from build123d import *

# Parameters (mm, degrees)
F1_DEPTH = 6.35


with BuildPart() as f1:
    # F0 (on Top) → F1 (new body)
    with BuildSketch(Plane.XY):
        with BuildLine():
            Line((-51.2445, 0), (-48.26, 0))
            ThreePointArc((-48.26, 0), (-54.61, 6.35), (-60.96, 0))
            Line((-60.96, 0), (-57.9755, 0))
            ThreePointArc((-57.9755, 0), (-54.61, 3.3655), (-51.2445, 0))
        make_face()
        with BuildLine():
            ThreePointArc((-60.96, 0), (-54.61, -6.35), (-48.26, 0))
            Line((-48.26, 0), (-51.2445, 0))
            ThreePointArc((-51.2445, 0), (-54.61, -3.3655), (-57.9755, 0))
            Line((-57.9755, 0), (-60.96, 0))
        make_face()
        with BuildLine():
            ThreePointArc((-34.1249732601, -34.1249732601), (-44.586426239, -18.4683024459), (-48.26, 0))
            ThreePointArc((-48.26, 0), (-54.61, -6.35), (-60.96, 0))
            ThreePointArc((-60.96, 0), (-37.1100967124, -48.3628196242), (15.7776089894, -58.8828383706))
            ThreePointArc((15.7776089894, -58.8828383706), (12.4119310117, -58.8612144651), (9.5300837025, -57.1224758622))
            ThreePointArc((9.5300837025, -57.1224758622), (-17.6688931256, -55.1507929201), (-40.9499679121, -40.9499679121))
            ThreePointArc((-40.9499679121, -40.9499679121), (-40.9499679121, -36.2802347291), (-36.2802347291, -36.2802347291))
            Line((-36.2802347291, -36.2802347291), (-34.1249732601, -34.1249732601))
        make_face()
        with BuildLine():
            ThreePointArc((8.1381651285, -50.6584754246), (9.8124734412, -48.096685942), (12.4906071166, -46.6155803767))
            ThreePointArc((12.4906071166, -46.6155803767), (-12.4906071166, -46.6155803767), (-34.1249732601, -34.1249732601))
            Line((-34.1249732601, -34.1249732601), (-36.2802347291, -36.2802347291))
            ThreePointArc((-36.2802347291, -36.2802347291), (-15.8011857696, -48.8142744725), (8.1381651285, -50.6584754246))
        make_face()
        with BuildLine():
            ThreePointArc((20.484108053, -52.7492093736), (17.9997431273, -47.7114156628), (12.4906071166, -46.6155803767))
            Line((12.4906071166, -46.6155803767), (13.2794875661, -49.5597222952))
            ThreePointArc((13.2794875661, -49.5597222952), (16.1442382916, -50.129556644), (17.436108053, -52.7492093736))
            ThreePointArc((17.436108053, -52.7492093736), (16.7537607827, -54.7593396122), (14.98872854, -55.9386964521))
            Line((14.98872854, -55.9386964521), (15.7776089894, -58.8828383706))
            ThreePointArc((15.7776089894, -58.8828383706), (19.1719017639, -56.6148444479), (20.484108053, -52.7492093736))
        make_face()
        with BuildLine():
            Line((13.2794875661, -49.5597222952), (12.4906071166, -46.6155803767))
            ThreePointArc((12.4906071166, -46.6155803767), (9.8124734412, -48.096685942), (8.1381651285, -50.6584754246))
            ThreePointArc((8.1381651285, -50.6584754246), (10.7229089499, -50.1749946453), (13.2794875661, -49.5597222952))
        make_face()
        with BuildLine():
            ThreePointArc((9.5300837025, -57.1224758622), (12.4119310117, -58.8612144651), (15.7776089894, -58.8828383706))
            Line((15.7776089894, -58.8828383706), (14.98872854, -55.9386964521))
            ThreePointArc((14.98872854, -55.9386964521), (12.2736861565, -56.5964342705), (9.5300837025, -57.1224758622))
        make_face()
    extrude(amount=-F1_DEPTH)


solid = f1.part
Check sheet for the modelled part. Datum: model origin and axes. Units: mm. Round coordinates to 2 decimals unless told otherwise and drop trailing zeros. Write each loop counter-clockwise with the first axis right and the second up, starting at its lowest first coordinate (ties: lowest second). Pieces come first, ordered by that corner, then holes. Notation, with made-up numbers: (8, 1) -> (14, 1) arc R15 ccw to (14, 18) -> close; hole circle Ø1 at (56, 21). An arc over 180 degrees is marked (long way). Answer as CSV lines item,"result". Start each with the question number.
1) Section check B-B on z = -3. Enter the section's corners in (x, y), and give its area (3 significant figures).
2) Section check D-D on y = -13. Enter the section's corners in (x, z).
3) Section check A-A on x = -23. Enter the section's corners in (y, z).
4) Section check C-C on x = 3. Enter the section's corners in (y, z), and give its area (3 significant figures).
5) Material ranges on line 1 (Y direction, x = -0.5, z = -2); line 2 (X direction, y = -36.5, z = -0.25); line 3 (X direction, y = -41, z = -3.75), recorded low to high. Write a range as from..to.
6) Go/stop test with flat-tipped pins: P1, Ø1.5, axis at y = -5.5, z = -3.5, coming from the +X side; P2, Ø3, axis at y = -9, z = -5, coming from the -X side; P3, Ø1, axis at y = -31.5, z = -2, coming from the -X side; P4, Ø5.5, axis at x = -54.61, y = 0, coming from the -Z side. Record where each tip stops, or that it passes through.
7) Release check for a two-part mould opening along Y. For faces 1 (the cylindrical face through (-54.47, 6.35, -3.13)), 2 (the cylindrical face through (-41, -36.33, -3.13)), 3 (the flat face through (-36, -35, -6.35)) record: pulls with the +Y half, pulls with the -Y half, needs draft (parallel to the pull), parting line crosses it, or undercut.
Found:
1,outline,"(-60.96, 0) arc R60.96 ccw to (15.78, -58.88) arc R6.35 ccw to (12.49, -46.62) arc R48.26 cw to (-48.26, 0) arc R6.35 ccw to start; hole circle Ø6.73 at (-54.61, 0); hole (-40.95, -40.95) arc R57.91 ccw to (14.99, -55.94) arc R3.3 ccw to (13.28, -49.56) arc R51.31 cw to (-36.28, -36.28) arc R3.3 ccw to start"
1,area,"950 mm^2"
2,outline,"(-59.56, -6.35) -> (-46.48, -6.35) -> (-46.48, 0) -> (-59.56, 0) -> close"
3,outline,"(-56.45, -6.35) -> (-53.15, -6.35) -> (-53.15, 0) -> (-56.45, 0) -> close; (-45.86, -6.35) -> (-42.43, -6.35) -> (-42.43, 0) -> (-45.86, 0) -> close"
4,outline,"(-60.89, -6.35) -> (-57.83, -6.35) -> (-57.83, 0) -> (-60.89, 0) -> close; (-51.22, -6.35) -> (-48.17, -6.35) -> (-48.17, 0) -> (-51.22, 0) -> close"
4,area,"38.8 mm^2"
5,line 1,"y = -60.96..-57.91, -51.31..-48.26"
5,line 2,"x = -48.82..-41.15, -36.06..-31.57"
5,line 3,"x = -45.11..-40.9, -30.85..-25.46"
6,P1,"stops at x = -47.85"
6,P2,"stops at x = -60.5"
6,P3,"stops at x = -52.49"
6,P4,"passes through"
7,face 1,"pulls with the +Y half"
7,face 2,"undercut"
7,face 3,"needs draft"
